from build123d import *

# Parameters (mm, degrees)
BOSS_EXTRUDE1_DEPTH     = 12.7
SKETCH5_W               = 5
SKETCH5_H               = 12.7
CUT_EXTRUDE2_DEPTH      = 1
CUT_EXTRUDE2_DEPTH_BACK = 39.1
SKETCH6_R               = 1.625
CUT_EXTRUDE3_DEPTH      = 13.7
FILLET1_R               = 2.54
FILLET2_R               = 0.762


with BuildPart() as part:
    # Sketch1 → Boss-Extrude1 (new body)
    with BuildSketch(Plane.XY):
        with BuildLine():
            Line((-4.75, -6.123225575), (-4.75, -10.16))
            Line((-4.75, -10.16), (-8.56, -10.16))
            Line((-8.56, -10.16), (-8.56, -8.128))
            Line((-8.56, -8.128), (-6.953663109, -8.128))
            Line((-6.953663109, -8.128), (-6.953663109, -6.745923719))
            ThreePointArc((-6.953663109, -6.745923719), (-9.212293425, 0.188355946), (-5.744562647, 6.604))
            Line((-5.744562647, 6.604), (-19.05, 6.604))
            Line((-19.05, 6.604), (-19.05, 21.104))
            Line((-19.05, 21.104), (19.05, 21.104))
            Line((19.05, 21.104), (19.05, 6.604))
            Line((19.05, 6.604), (5.744562647, 6.604))
            ThreePointArc((5.744562647, 6.604), (9.212293425, 0.188355946), (6.953663109, -6.745923719))
            Line((6.953663109, -6.745923719), (6.953663109, -8.128))
            Line((6.953663109, -8.128), (8.56, -8.128))
            Line((8.56, -8.128), (8.56, -10.16))
            Line((8.56, -10.16), (4.75, -10.16))
            Line((4.75, -10.16), (4.75, -6.123225575))
            ThreePointArc((4.75, -6.123225575), (0, 6.604), (-4.75, -6.123225575))
        make_face()
    extrude(amount=BOSS_EXTRUDE1_DEPTH)

    # Sketch5 → Cut-Extrude2 (cut, two sides)
    with BuildSketch(Plane.ZY.offset(19.05)) as cut_extrude2_sk:
        with Locations((6.35, 14.754)):
            Rectangle(SKETCH5_W, SKETCH5_H)
    extrude(amount=CUT_EXTRUDE2_DEPTH, mode=Mode.SUBTRACT)
    extrude(cut_extrude2_sk.sketch, amount=-CUT_EXTRUDE2_DEPTH_BACK, mode=Mode.SUBTRACT)

    # Sketch6 → Cut-Extrude3 (cut, through all)
    with BuildSketch(Plane.XY.offset(12.7)):
        with Locations((-10.16, 14.754)):
            Circle(SKETCH6_R)
        with Locations((10.16, 14.754)):
            Circle(SKETCH6_R)
    extrude(amount=-CUT_EXTRUDE3_DEPTH, mode=Mode.SUBTRACT)

    # Fillet1
    fillet1_edges = [part.edges().sort_by_distance(p)[0] for p in [
        (4.75, -10.16, 6.35),
        (4.75, -6.123225575, 6.35),
        (-4.75, -6.123225575, 6.35),
        (-4.75, -10.16, 6.35),
    ]]
    fillet(fillet1_edges, radius=FILLET1_R)

    # Fillet2
    fillet2_edges = [part.edges().sort_by_distance(p)[0] for p in [
        (-8.56, -8.128, 6.35),
        (-6.953663109, -8.128, 6.35),
        (-6.953663109, -6.745923719, 6.35),
        (-5.744562647, 6.604, 6.35),
        (5.744562647, 6.604, 6.35),
        (6.953663109, -6.745923719, 6.35),
        (6.953663109, -8.128, 6.35),
        (8.56, -8.128, 6.35),
        (8.56, -10.16, 6.35),
        (-8.56, -10.16, 6.35),
    ]]
    fillet(fillet2_edges, radius=FILLET2_R)


solid = part.part
Work out the finished part from the listing and answer in its coordinate system (mm). A direction names the side the tool comes from. Give positions to 0.01 mm unless a question says otherwise; leave off trailing zeros. Write each loop counter-clockwise with the first axis right and the second up, starting at its lowest first coordinate (ties: lowest second). Pieces come first, ordered by that corner, then holes. Notation, with made-up numbers: (-32, 86) - (-4, 86) arc R18 cw to (-4, 113) - close; hole circle Ø8 at (77, 18). An arc over 180 degrees is marked (long way). One line per item, written item: value. Start each with the question number.
1. For faces 1 (the flat face through (0, 8.404, 6)), 2 (the flat face through (0, 21.104, 11)), 3 (the cylindrical face through (5.474, -9.396, 6.439)), 4 (the cylindrical face through (-4.91, -6.29, 6.44)), determine the directions among +Z, -Z, +X, -X, +Y, -Y from which every point of the face is accessible in a straight line to the end or side of a thin tool.
2. Find section B-B (y = 9). Write down the section's boundary in (x, z), then the cut area to 3 significant figures.
3. Find section D-D (x = 0). Write down the section's boundary in (y, z).
4. Given pin 1 (1.9 mm diameter, centred on x = 10.16, y = 14.754, fed in from -Z); pin 2 (3.5 mm diameter, centred on x = -14.5, z = 7, fed in from -Y); pin 3 (4 mm diameter, centred on x = 0.5, z = 8, fed in from +Y); pin 4 (1 mm diameter, centred on y = -1.5, z = 7, fed in from +X), each flat-ended and moving along its own axis, determine where each tip first touches the part or whether it passes through.
5. For a pull along X with two mould halves and no side action, classify faces 5 (the flat face through (-19.05, 14, 3)), 6 (the cylindrical face through (0.2, 6.6, 6.3)), 7 (the flat face through (0, 15, 3.85)) as +X half, -X half, draft (parallel to the pull), parting line (faces both ways), or undercut.
6. Find section A-A (x = 10.16). Write down the section's boundary in (y, z).
7. Find section C-C (z = 9.75). State how many separate pieces and enclosed holes the cut face has, then the cut area to 3 significant figures.
8. Consider probe 1 along Z at (x, y) = (-13.5, 15); probe 2 along Y at (x, z) = (-10.16, 11.8); probe 3 along X at (y, z) = (16, 10). Determine where each line is inside the solid, lowest interval first.
Geometry results:
1. face 1: +X, -X, +Y
1. face 2: +Z, -Z, +X, -X, +Y
1. face 3: +Z, -Z, -Y
1. face 4: +Z, -Z
2. outline: (-19.05, 0) - (19.05, 0) - (19.05, 3.85) - (-19.05, 3.85) - close; (-19.05, 8.85) - (19.05, 8.85) - (19.05, 12.7) - (-19.05, 12.7) - close
2. area: 293 mm2
3. outline: (6.6, 0) - (21.1, 0) - (21.1, 3.85) - (8.4, 3.85) - (8.4, 8.85) - (21.1, 8.85) - (21.1, 12.7) - (6.6, 12.7) - close
4. pin 1: through
4. pin 2: y = 6.6
4. pin 3: y = 21.1
4. pin 4: x = 9.24
5. face 5: -X half
5. face 6: undercut
5. face 7: draft
6. outline: (6.6, 0) - (13.13, 0) - (13.13, 3.85) - (8.4, 3.85) - (8.4, 8.85) - (13.13, 8.85) - (13.13, 12.7) - (6.6, 12.7) - close; (16.38, 0) - (21.1, 0) - (21.1, 3.85) - (16.38, 3.85) - close; (16.38, 8.85) - (21.1, 8.85) - (21.1, 12.7) - (16.38, 12.7) - close
7. separate pieces: 1
7. enclosed holes: 2
7. area: 619 mm2
8. probe 1: 0 to 3.85, 8.85 to 12.7
8. probe 2: 6.6 to 13.13, 16.38 to 21.1
8. probe 3: -19.05 to -11.2, -9.12 to 9.12, 11.2 to 19.05
